Check sheet for the modelled part. Datum: model origin and axes. Units: mm. Face numbers are marked on the shaded views. Give positions to 0.01 mm unless a question says otherwise; leave off trailing zeros. Order: outer loops, then holes, each group sorted by start corner. A loop starts at its lowest first (then second) coordinate and runs counter-clockwise, first axis right, second up. Notation, with made-up numbers: (42, 56.5) - (48, 56.5) arc R13 cw to (48, 72.5) - close; hole circle Ø5 at (-6, 83). An arc over 180 degrees is marked (long way). Answer in a Markdown table with one row per item.
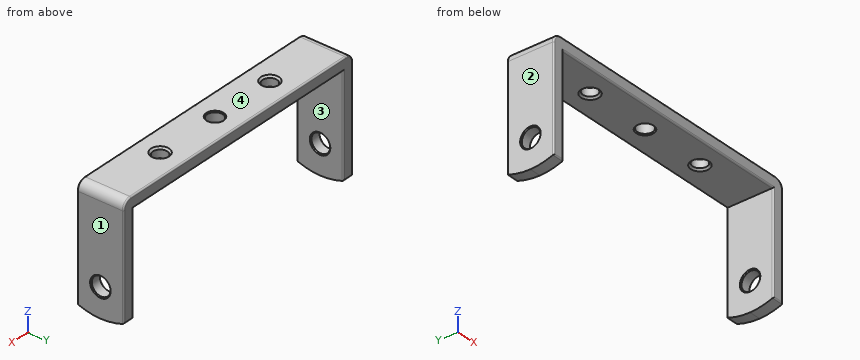
from build123d import *

# Parameters (mm, degrees)
F1_DEPTH = 25.4
F2_R     = 5.08
F3_DEPTH = 152.401
F4_R     = 3.937
F4_R_2   = 4.2545
F5_DEPTH = 63.501
F6_SIZE  = 1.016
F7_SIZE  = 0.508
F8_R     = 4.826
F9_R     = 0.762


with BuildPart() as f1:
    # F0 (on Front) → F1 (new body)
    with BuildSketch(Plane.XZ):
        Polygon((-69.85, -57.15), (-69.85, 0), (0, 0), (69.85, 0), (69.85, -57.15), (76.2, -57.15), (76.2, 6.35), (0, 6.35), (-76.2, 6.35), (-76.2, -57.15), align=None)
    extrude(amount=F1_DEPTH)

    # F2 (on face) → F3 (cut, through all)
    with BuildSketch(Plane(origin=(-76.2, 0, 0), x_dir=(0, -1, 0), z_dir=(-1, 0, 0))):
        with Locations((12.7, -41.275)):
            Circle(F2_R)
        with BuildLine():
            ThreePointArc((25.4, -54.7590686819), (19.1615507536, -56.5470626836), (12.7, -57.15))
            Line((12.7, -57.15), (25.4, -57.15))
            Line((25.4, -57.15), (25.4, -54.7590686819))
        make_face()
        with BuildLine():
            ThreePointArc((12.7, -57.15), (6.2384492464, -56.5470626836), (0, -54.7590686819))
            Line((0, -54.7590686819), (0, -57.15))
            Line((0, -57.15), (12.7, -57.15))
        make_face()
    extrude(amount=-F3_DEPTH, mode=Mode.SUBTRACT)

    # F4 (on face) → F5 (cut, through all)
    with BuildSketch(Plane.XY.offset(6.35)):
        with Locations((-36.5125, -12.7)):
            Circle(F4_R)
        with Locations((0, -12.7)):
            Circle(F4_R_2)
        with Locations((36.5125, -12.7)):
            Circle(F4_R)
    extrude(amount=-F5_DEPTH, mode=Mode.SUBTRACT)

    # F6
    f6_edges = [f1.edges().sort_by_distance(p)[0] for p in [
        (-40.4495, -12.7, 6.35),
        (32.5755, -12.7, 6.35),
        (32.5755, -12.7, 0),
        (-40.4495, -12.7, 0),
    ]]
    chamfer(f6_edges, length=F6_SIZE)

    # F7
    f7_edges = [f1.edges().sort_by_distance(p)[0] for p in [
        (-4.2545, -12.7, 6.35),
        (-4.2545, -12.7, 0),
        (-69.85, -7.62, -41.275),
        (69.85, -7.62, -41.275),
        (76.2, -7.62, -41.275),
        (-76.2, -7.62, -41.275),
    ]]
    chamfer(f7_edges, length=F7_SIZE)

    # F8
    f8_edges = [f1.edges().sort_by_distance(p)[0] for p in [
        (-76.2, -12.7, 6.35),
        (76.2, -12.7, 6.35),
    ]]
    fillet(f8_edges, radius=F8_R)

    # F9
    f9_edges = [f1.edges().sort_by_distance(p)[0] for p in [
        (0, -25.4, 6.35),
        (-73.025, -25.4, -54.759069),
        (-69.85, -25.4, -27.379534),
        (0, -25.4, 0),
        (69.85, -25.4, -27.379534),
        (73.025, -25.4, -54.759069),
        (0, 0, 6.35),
        (69.85, 0, -27.379534),
        (0, 0, 0),
        (-69.85, 0, -27.379534),
        (73.025, 0, -54.759069),
        (-73.025, 0, -54.759069),
    ]]
    fillet(f9_edges, radius=F9_R)


solid = f1.part
(1) Cross-section at C-C, the plane x = 44. Record the cut outline in (y, z).
Geometry says:
| item | result |
|---|---|
| outline | (-25.4, 0.76) arc R0.76 ccw to (-24.64, 0) - (-0.76, 0) arc R0.76 ccw to (0, 0.76) - (0, 5.59) arc R0.76 ccw to (-0.76, 6.35) - (-24.64, 6.35) arc R0.76 ccw to (-25.4, 5.59) - close |
(2) Mould release check, pull along X, two halves, no side actions. Record for the marked faces 1, 2, 3 and 4: pulls with the +X half, pulls with the -X half, needs draft (parallel to the pull), parting line crosses it, or undercut.
Geometry says:
| item | result |
|---|---|
| face 1 | pulls with the +X half |
| face 2 | pulls with the -X half |
| face 3 | undercut |
| face 4 | needs draft |
(3) Cross-section at B-B, the plane x = 0. Record the cut outline in (y, z), then the cut area to 3 significant figures.
Geometry says:
| item | result |
|---|---|
| outline | (-25.4, 0.76) arc R0.76 ccw to (-24.64, 0) - (-17.46, 0) - (-16.95, 0.51) - (-16.95, 5.84) - (-17.46, 6.35) - (-24.64, 6.35) arc R0.76 ccw to (-25.4, 5.59) - close; (-8.45, 0.51) - (-7.94, 0) - (-0.76, 0) arc R0.76 ccw to (0, 0.76) - (0, 5.59) arc R0.76 ccw to (-0.76, 6.35) - (-7.94, 6.35) - (-8.45, 5.84) - close |
| area | 106 mm² |
(4) Cross-section at D-D, the plane y = -5.5. Record the cut outline in (x, z).
Geometry says:
| item | result |
|---|---|
| outline | (-76.2, -56.4) - (-69.85, -56.4) - (-69.85, 0) - (69.85, 0) - (69.85, -56.4) - (76.2, -56.4) - (76.2, 1.52) arc R4.83 ccw to (71.37, 6.35) - (-71.37, 6.35) arc R4.83 ccw to (-76.2, 1.52) - close |
(5) Cross-section at A-A, the plane z = -8. Record the cut outline in (x, y).
Geometry says:
| item | result |
|---|---|
| outline | (-76.2, -24.64) arc R0.76 ccw to (-75.44, -25.4) - (-70.61, -25.4) arc R0.76 ccw to (-69.85, -24.64) - (-69.85, -0.76) arc R0.76 ccw to (-70.61, 0) - (-75.44, 0) arc R0.76 ccw to (-76.2, -0.76) - close; (69.85, -24.64) arc R0.76 ccw to (70.61, -25.4) - (75.44, -25.4) arc R0.76 ccw to (76.2, -24.64) - (76.2, -0.76) arc R0.76 ccw to (75.44, 0) - (70.61, 0) arc R0.76 ccw to (69.85, -0.76) - close |
(6) Gauge pin test, flat ends, axial feed: P1, Ø12.5, axis at x = -36.51, y = -12.7, coming from the +Z side; P2, Ø7, axis at x = 36.51, y = -12.7, coming from the -Z side. Record the tip position at first contact, or that the pin passes through.
Geometry says:
| item | result |
|---|---|
| P1 | z = 6.35 |
| P2 | through |
(7) Thickness scan on L1, parallel to X at y = -9.5, z = -6; L2, parallel to Z at x = -71.65, y = -12.7 (3 decimals); L3, parallel to Z at x = -74.3, y = -12.7 (3 decimals). Record the ranges inside material, lowest first.
Geometry says:
| item | result |
|---|---|
| L1 | -76.2 to -69.85, 69.85 to 76.2 |
| L2 | -57.15 to -46.355, -36.195 to 6.342 |
| L3 | -57.15 to -46.355, -36.195 to 5.362 |
